from build123d import *

# Parameters (mm, degrees)
MODEL_W                 = 3
MODEL_H                 = 3
SALIENTE_EXTRUIR1_DEPTH = 3


with BuildPart() as part:
    # Model → Saliente-Extruir1 (new body)
    with BuildSketch(Plane.XY):
        with BuildLine():
            Line((9.904781567, 296.774995526), (108.904781567, 296.774995526))
            ThreePointArc((108.904781567, 296.774995526), (113.404781567, 292.274995526), (108.904781567, 287.774995526))
            Line((108.904781567, 287.774995526), (9.904781567, 287.774995526))
            ThreePointArc((9.904781567, 287.774995526), (5.404781567, 292.274995526), (9.904781567, 296.774995526))
        make_face()
        with Locations((9.904781567, 292.274995526)):
            Rectangle(MODEL_W, MODEL_H, mode=Mode.SUBTRACT)
        with Locations((18.904781567, 292.274995526)):
            Rectangle(MODEL_W, MODEL_H, mode=Mode.SUBTRACT)
        with Locations((27.904781567, 292.274995526)):
            Rectangle(MODEL_W, MODEL_H, mode=Mode.SUBTRACT)
        with Locations((36.904781567, 292.274995526)):
            Rectangle(MODEL_W, MODEL_H, mode=Mode.SUBTRACT)
        with Locations((45.904781567, 292.274995526)):
            Rectangle(MODEL_W, MODEL_H, mode=Mode.SUBTRACT)
        with Locations((54.904781567, 292.274995526)):
            Rectangle(MODEL_W, MODEL_H, mode=Mode.SUBTRACT)
        with Locations((63.904781567, 292.274995526)):
            Rectangle(MODEL_W, MODEL_H, mode=Mode.SUBTRACT)
        with Locations((72.904781567, 292.274995526)):
            Rectangle(MODEL_W, MODEL_H, mode=Mode.SUBTRACT)
        with Locations((81.904781567, 292.274995526)):
            Rectangle(MODEL_W, MODEL_H, mode=Mode.SUBTRACT)
        with Locations((90.904781567, 292.274995526)):
            Rectangle(MODEL_W, MODEL_H, mode=Mode.SUBTRACT)
        with Locations((108.904781567, 292.274995526)):
            Rectangle(MODEL_W, MODEL_H, mode=Mode.SUBTRACT)
        with Locations((99.904781567, 292.274995526)):
            Rectangle(MODEL_W, MODEL_H, mode=Mode.SUBTRACT)
    extrude(amount=SALIENTE_EXTRUIR1_DEPTH)


solid = part.part
For this review, take the finished solid that the model builds, in its own axes (mm). Coordinates: 2 decimals unless noted, no trailing zeros. Order: outer loops, then holes, each group sorted by start corner. A loop starts at its lowest first (then second) coordinate and runs counter-clockwise, first axis right, second up. Notation, with made-up numbers: (59, 82.25) - (70, 82.25) arc R5 ccw to (70, 87.25) - close; hole circle Ø5 at (80, 46.25). An arc over 180 degrees is marked (long way). Use one line per item in the form item = value.
Q1. Draft analysis for pull direction Y (two halves, no side actions). For faces 1 (the flat face through (59, 296.775, 1)), 2 (the flat face through (60, 292, 0)), 3 (the flat face through (100, 290.775, 1)), state which applies: +Y half, -Y half, draft (parallel to the pull), parting line (faces both ways), or undercut.
Checked values:
face_1 = +Y half
face_2 = draft
face_3 = undercut
Q2. Consider section B-B (z = 1.4). Give the number of separate pieces and of enclosed holes in the cut face, then the cut area to 3 significant figures.
Checked values:
separate_pieces = 1
enclosed_holes = 12
area = 847 mm2
Q3. Consider section A-A (x = 46). Give the boundary of the cut face in (y, z) (3 decimals).
Checked values:
outline = (287.775, 0) - (290.775, 0) - (290.775, 3) - (287.775, 3) - close; (293.775, 0) - (296.775, 0) - (296.775, 3) - (293.775, 3) - close
Q4. For P1, Ø1.5, axis at y = 290, z = 1, coming from the +X side, flat-tipped, find the tip position at first contact; note if it passes through.
Checked values:
P1 = 113.14
Q5. For probe 1 along Y at (x, z) = (20, 2.4) (3 decimals); probe 2 along X at (y, z) = (295.5, 2.75); probe 3 along X at (y, z) = (296, 1.4), list the stretches that pass through material, from the lowest coordinate up. Write a range as from..to.
Checked values:
probe_1 = 287.775..290.775, 293.775..296.775
probe_2 = 6.77..112.04
probe_3 = 7.38..111.43
Q6. Consider section C-C (y = 295.5). Give the boundary of the cut face in (x, z).
Checked values:
outline = (6.77, 0) - (112.04, 0) - (112.04, 3) - (6.77, 3) - close
